Input: part model. Units: mm. Frame: model coordinates. Face numbers are marked on the shaded views. A direction names the side the tool comes from. Give positions to 0.01 mm unless a question says otherwise; leave off trailing zeros. Loops run counter-clockwise (first coordinate to the right, second up) from the corner with the lowest first, then second, coordinate; pieces in that order, holes last. Notation, with made-up numbers: M -18,77 L 18,77 A31 ccw 18,106 Z; hole C -20.5,43.25 d6. An arc over 180 degrees is marked long. Answer as a JSON object with one key per item and string values. Group by question number.
1) Ray query, L1, parallel to X at y = 48, z = 45; L2, parallel to X at y = -2, z = -17; L3, parallel to X at y = 9, z = 34. Return the intervals inside material, ascending.
2) Section query B-B on y = 15. Return loops of the section in (x, z).
3) Access query for the marked faces 4, 5, 6 and 7. Directions: +Z, -Z, +X, -X, +Y, -Y. A direction counts if a zero-diameter tool reaches every point of the face in a straight line with its end or side. Return the directions, or none.
4) First-contact query: P1, Ø6, axis at y = 74, z = -12.5, coming from the -X side; P2, Ø5.5, axis at x = 25, z = 12.5, coming from the -Y side; P3, Ø5.5, axis at x = 12.5, z = 25, coming from the +Y side. Flat tips, straight axial feed; report the tip coordinate or a pass-through.
5) Section query A-A on y = 82. Count the separate pieces of the cut face and the enclosed holes in it, plus the area to 3 significant figures.
6) Draft query along X for the marked faces 1, 2 and 3. Return one class per face: +X half, -X half, draft (parallel to the pull), parting line (faces both ways), or undercut.
from build123d import *

# Parameters (mm, degrees)
SKETCH_1_R               = 50
EXTRUDE_1_DEPTH          = 80
FILLET_1_R               = 2
SKETCH_2_R               = 5.5
CUT_EXTRUDE_1_DEPTH      = 80
SKETCH_3_W               = 11.906162192
SKETCH_3_H               = 92.178298694
CUT_EXTRUDE_2_DEPTH      = 4
SKETCH_4_W               = 11.810184272
SKETCH_4_H               = 42.447784179
CUT_EXTRUDE_3_DEPTH      = 10
SKETCH_5_W               = 11.942044514
SKETCH_5_H               = 45.487816108
CUT_EXTRUDE_4_DEPTH      = 10
SKETCH_6_W               = 11.810184272
SKETCH_6_H               = 60.078318052
CUT_EXTRUDE_5_DEPTH      = 20
CUT_EXTRUDE_7_DEPTH      = 50
FILLET_2_R               = 2
SKETCH_8_R               = 50
EXTRUDE_2_DEPTH          = 90
SKETCH_9_R               = 50
EXTRUDE_3_DEPTH          = 100
FILLET_3_R               = 2
SKETCH_10_R              = 15
CUT_EXTRUDE_8_DEPTH      = 100
SKETCH_11_R              = 3
CUT_EXTRUDE_9_DEPTH      = 10
PATTERN_CIRCULAR_1_COUNT = 4
SKETCH_12_R              = 3
CUT_EXTRUDE_10_DEPTH     = 10
PATTERN_CIRCULAR_2_COUNT = 4
SKETCH_13_R              = 2
CUT_EXTRUDE_11_DEPTH     = 10
PATTERN_CIRCULAR_3_COUNT = 4
SKETCH_14_R              = 2
CUT_EXTRUDE_12_DEPTH     = 10


with BuildPart() as part:
    # 草图1 → 凸台-拉伸1 (new body)
    with BuildSketch(Plane(origin=(0, 0, 0), x_dir=(1, 0, 0), z_dir=(0, 1, 0))):
        Polygon((-59.119808165, 53.642938728), (52.826892357, 53.642938728), (52.826892357, -53.523119778), (-59.119808165, -53.523119778), (-59.119808165, -72.079800299), (-127.882584058, -72.079800299), (-127.882584058, -25.63201612), (-59.119808165, -25.63201612), align=None)
        Circle(SKETCH_1_R, mode=Mode.SUBTRACT)
    extrude(amount=EXTRUDE_1_DEPTH)

    # 圆角1
    fillet_1_edges = [part.edges().sort_by_distance(p)[0] for p in [
        (-93.501196111, 0, 25.63201612),
        (-93.501196111, 80, 72.079800299),
        (-59.119808165, 40, -53.642938728),
        (52.826892357, 40, -53.642938728),
        (52.826892357, 40, 53.523119778),
        (-127.882584058, 40, 25.63201612),
        (-93.501196111, 80, 25.63201612),
        (-93.501196111, 0, 72.079800299),
    ]]
    fillet(fillet_1_edges, radius=FILLET_1_R)

    # 草图2 → 切除-拉伸1 (cut)
    with BuildSketch(Plane(origin=(0, 80, 0), x_dir=(1, 0, 0), z_dir=(0, 1, 0))):
        with Locations((-48.119582726, 44.979282561)):
            Circle(SKETCH_2_R)
        with Locations((42.826400195, 44.979282561)):
            Circle(SKETCH_2_R)
        with Locations((42.826400195, -44.420910434)):
            Circle(SKETCH_2_R)
    extrude(amount=-CUT_EXTRUDE_1_DEPTH, mode=Mode.SUBTRACT)

    # 草图3 → 切除-拉伸2 (cut)
    with BuildSketch(Plane.XY.offset(72.079800299)):
        with Locations((-76.966233581, 38.147560985)):
            Rectangle(SKETCH_3_W, SKETCH_3_H)
    extrude(amount=-CUT_EXTRUDE_2_DEPTH, mode=Mode.SUBTRACT)

    # 草图4 → 切除-拉伸3 (cut)
    with BuildSketch(Plane(origin=(0, 80, 0), x_dir=(1, 0, 0), z_dir=(0, 1, 0))):
        with Locations((-77.014222541, -46.85590821)):
            Rectangle(SKETCH_4_W, SKETCH_4_H)
    extrude(amount=-CUT_EXTRUDE_3_DEPTH, mode=Mode.SUBTRACT)

    # 草图5 → 切除-拉伸4 (cut)
    with BuildSketch(Plane.XZ):
        with Locations((-76.94829242, 45.335892245)):
            Rectangle(SKETCH_5_W, SKETCH_5_H)
    extrude(amount=-CUT_EXTRUDE_4_DEPTH, mode=Mode.SUBTRACT)

    # 草图6 → 切除-拉伸5 (cut)
    with BuildSketch(Plane(origin=(0, 0, 25.63201612), x_dir=(-1, 0, 0), z_dir=(0, 0, -1))):
        with Locations((77.014222541, 39.960840974)):
            Rectangle(SKETCH_6_W, SKETCH_6_H)
    extrude(amount=-CUT_EXTRUDE_5_DEPTH, mode=Mode.SUBTRACT)

    # 草图7 → 切除-拉伸7 (cut)
    with BuildSketch(Plane(origin=(0, 0, 25.63201612), x_dir=(-1, 0, 0), z_dir=(0, 0, -1))):
        Polygon((125.882584058, 41.670977544), (82.919314677, 41.670977544), (82.919314677, 38.149415643), (125.882584058, 38.149415643), (132.648981097, 38.149415643), (132.648981097, 41.670977544), align=None)
    extrude(amount=-CUT_EXTRUDE_7_DEPTH, mode=Mode.SUBTRACT)

    # 圆角2
    fillet_2_edges = [part.edges().sort_by_distance(p)[0] for p in [
        (-127.882584058, 38.149415643, 49.855908209),
        (-127.882584058, 41.670977544, 49.855908209),
        (-104.400949368, 38.149415643, 25.63201612),
        (-104.400949368, 41.670977544, 25.63201612),
        (-127.29679762, 38.149415643, 26.217802557),
        (-127.29679762, 41.670977544, 26.217802557),
    ]]
    fillet(fillet_2_edges, radius=FILLET_2_R)

    # 草图8 → 凸台-拉伸2 (add)
    with BuildSketch(Plane(origin=(0, 0, 0), x_dir=(1, 0, 0), z_dir=(0, 1, 0))):
        Circle(SKETCH_8_R)
    extrude(amount=EXTRUDE_2_DEPTH)

    # 草图9 → 凸台-拉伸3 (add)
    with BuildSketch(Plane(origin=(0, 90, 0), x_dir=(1, 0, 0), z_dir=(0, 1, 0))):
        Circle(SKETCH_9_R)
    extrude(amount=-EXTRUDE_3_DEPTH)

    # 圆角3
    fillet_3_edges = [part.edges().sort_by_distance(p)[0] for p in [
        (-50, 90, 0),
        (-50, -10, 0),
    ]]
    fillet(fillet_3_edges, radius=FILLET_3_R)

    # 草图10 → 切除-拉伸8 (cut)
    with BuildSketch(Plane.XZ.offset(10)):
        Circle(SKETCH_10_R)
    extrude(amount=-CUT_EXTRUDE_8_DEPTH, mode=Mode.SUBTRACT)

    # 草图11 → 切除-拉伸9 (cut)
    with BuildSketch(Plane.XZ.offset(10)):
        with Locations((25, 0)):
            Circle(SKETCH_11_R)
        with Locations((25, 12.5)):
            Circle(SKETCH_11_R)
        with Locations((25, -12.5)):
            Circle(SKETCH_11_R)
    cut_extrude_9 = extrude(amount=-CUT_EXTRUDE_9_DEPTH, mode=Mode.SUBTRACT)

    # 阵列(圆周)1: 切除-拉伸9 ×4 about axis
    pattern_circular_1_axis = Axis((0, 0, 0), (0, 1, 0))
    for i in range(1, PATTERN_CIRCULAR_1_COUNT):
        add(cut_extrude_9.rotate(pattern_circular_1_axis, i * 360 / PATTERN_CIRCULAR_1_COUNT), mode=Mode.SUBTRACT)

    # 草图12 → 切除-拉伸10 (cut)
    with BuildSketch(Plane(origin=(0, 90, 0), x_dir=(1, 0, 0), z_dir=(0, 1, 0))):
        with Locations((-12.5, 25)):
            Circle(SKETCH_12_R)
        with Locations((0, 25)):
            Circle(SKETCH_12_R)
        with Locations((12.5, 25)):
            Circle(SKETCH_12_R)
    cut_extrude_10 = extrude(amount=-CUT_EXTRUDE_10_DEPTH, mode=Mode.SUBTRACT)

    # 阵列(圆周)2: 切除-拉伸10 ×4 about axis
    pattern_circular_2_axis = Axis((0, 0, 0), (0, 1, 0))
    for i in range(1, PATTERN_CIRCULAR_2_COUNT):
        add(cut_extrude_10.rotate(pattern_circular_2_axis, i * 360 / PATTERN_CIRCULAR_2_COUNT), mode=Mode.SUBTRACT)

    # 草图13 → 切除-拉伸11 (cut)
    with BuildSketch(Plane.XZ.offset(10)):
        with Locations((17, 17)):
            Circle(SKETCH_13_R)
    cut_extrude_11 = extrude(amount=-CUT_EXTRUDE_11_DEPTH, mode=Mode.SUBTRACT)

    # 阵列(圆周)3: 切除-拉伸11 ×4 about axis
    pattern_circular_3_axis = Axis((0, 0, 0), (0, 1, 0))
    for i in range(1, PATTERN_CIRCULAR_3_COUNT):
        add(cut_extrude_11.rotate(pattern_circular_3_axis, i * 360 / PATTERN_CIRCULAR_3_COUNT), mode=Mode.SUBTRACT)

    # 草图14 → 切除-拉伸12 (cut)
    with BuildSketch(Plane(origin=(0, 90, 0), x_dir=(1, 0, 0), z_dir=(0, 1, 0))):
        with Locations((-17, -17)):
            Circle(SKETCH_14_R)
        with Locations((-17, 17)):
            Circle(SKETCH_14_R)
        with Locations((17, 17)):
            Circle(SKETCH_14_R)
        with Locations((17, -17)):
            Circle(SKETCH_14_R)
    extrude(amount=-CUT_EXTRUDE_12_DEPTH, mode=Mode.SUBTRACT)


solid = part.part
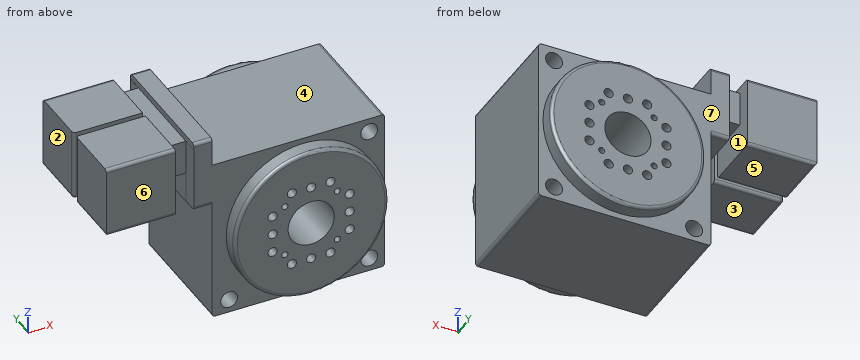
Output:
{
 "1": {"L1": "x = -127.88 to -82.92, -71.11 to 37.36, 48.3 to 52.83", "L2": "x = -47.02 to -19, -15 to 15, 19 to 47.02", "L3": "x = -127.88 to -82.92, -70.98 to 52.83"},
 "2": {"outline": "M -127.88,27.63 A2 ccw -125.88,25.63 L -82.92,25.63 L -82.92,45.63 L -71.11,45.63 L -71.11,25.63 L -59.12,25.63 L -59.12,-51.64 A2 ccw -57.12,-53.64 L 50.83,-53.64 A2 ccw 52.83,-51.64 L 52.83,51.52 A2 ccw 50.83,53.52 L -59.12,53.52 L -59.12,72.08 L -71.01,72.08 L -71.01,68.08 L -82.92,68.08 L -82.92,72.08 L -127.88,72.08 Z; hole C -48.12,-44.98 d11; hole C 0,0 d30; hole C 42.83,-44.98 d11; hole C 42.83,44.42 d11"},
 "3": {"face 4": "+Z, +X, +Y, -Y", "face 5": "-Z, -X, +Y, -Y", "face 6": "+Z, -Z, -X, -Y", "face 7": "+Y"},
 "4": {"P1": "stops at x = -59.12", "P2": "stops at y = 0", "P3": "stops at y = 80"},
 "5": {"separate pieces": "1", "enclosed holes": "17", "area": "6,760 mm^2"},
 "6": {"face 1": "undercut", "face 2": "-X half", "face 3": "draft"}
}
